from build123d import *

# Parameters (mm, degrees)
SKETCH1_R           = 3.25
SKETCH1_R_2         = 1.5
BOSS_EXTRUDE1_DEPTH = 10


with BuildPart() as part:
    # Sketch1 → Boss-Extrude1 (new body)
    with BuildSketch(Plane(origin=(0, 0, 0), x_dir=(1, 0, 0), z_dir=(0, 1, 0))):
        with BuildLine():
            Line((-40, -26.25), (40, -26.25))
            ThreePointArc((40, -26.25), (44.419417382, -24.419417382), (46.25, -20))
            Line((46.25, -20), (46.25, 20))
            ThreePointArc((46.25, 20), (44.419417382, 24.419417382), (40, 26.25))
            Line((40, 26.25), (-40, 26.25))
            ThreePointArc((-40, 26.25), (-44.419417382, 24.419417382), (-46.25, 20))
            Line((-46.25, 20), (-46.25, -20))
            ThreePointArc((-46.25, -20), (-44.419417382, -24.419417382), (-40, -26.25))
        make_face()
        with Locations((-40, 20)):
            Circle(SKETCH1_R, mode=Mode.SUBTRACT)
        with Locations((-40, -20)):
            Circle(SKETCH1_R, mode=Mode.SUBTRACT)
        with Locations((40, -20)):
            Circle(SKETCH1_R, mode=Mode.SUBTRACT)
        with Locations((40, 20)):
            Circle(SKETCH1_R, mode=Mode.SUBTRACT)
        with Locations((-43.78036994, 13.234550782)):
            Circle(SKETCH1_R_2, mode=Mode.SUBTRACT)
        with Locations((-39.934701703, 12.250275093)):
            Circle(SKETCH1_R_2, mode=Mode.SUBTRACT)
        with Locations((-36.10616509, 13.299212756)):
            Circle(SKETCH1_R_2, mode=Mode.SUBTRACT)
        with Locations((-33.299212756, 16.10616509)):
            Circle(SKETCH1_R_2, mode=Mode.SUBTRACT)
        with Locations((-32.250275093, 19.934701703)):
            Circle(SKETCH1_R_2, mode=Mode.SUBTRACT)
        with Locations((-33.234550782, 23.78036994)):
            Circle(SKETCH1_R_2, mode=Mode.SUBTRACT)
        with Locations((-33.234550782, -23.78036994)):
            Circle(SKETCH1_R_2, mode=Mode.SUBTRACT)
        with Locations((-32.250275093, -19.934701703)):
            Circle(SKETCH1_R_2, mode=Mode.SUBTRACT)
        with Locations((-33.299212756, -16.10616509)):
            Circle(SKETCH1_R_2, mode=Mode.SUBTRACT)
        with Locations((-36.10616509, -13.299212756)):
            Circle(SKETCH1_R_2, mode=Mode.SUBTRACT)
        with Locations((-39.934701703, -12.250275093)):
            Circle(SKETCH1_R_2, mode=Mode.SUBTRACT)
        with Locations((-43.78036994, -13.234550782)):
            Circle(SKETCH1_R_2, mode=Mode.SUBTRACT)
        with Locations((33.234550782, 23.78036994)):
            Circle(SKETCH1_R_2, mode=Mode.SUBTRACT)
        with Locations((32.250275093, 19.934701703)):
            Circle(SKETCH1_R_2, mode=Mode.SUBTRACT)
        with Locations((33.299212756, 16.10616509)):
            Circle(SKETCH1_R_2, mode=Mode.SUBTRACT)
        with Locations((39.934701703, 12.250275093)):
            Circle(SKETCH1_R_2, mode=Mode.SUBTRACT)
        with Locations((43.78036994, 13.234550782)):
            Circle(SKETCH1_R_2, mode=Mode.SUBTRACT)
        with Locations((36.10616509, 13.299212756)):
            Circle(SKETCH1_R_2, mode=Mode.SUBTRACT)
        with Locations((33.234550782, -23.78036994)):
            Circle(SKETCH1_R_2, mode=Mode.SUBTRACT)
        with Locations((32.250275093, -19.934701703)):
            Circle(SKETCH1_R_2, mode=Mode.SUBTRACT)
        with Locations((33.299212756, -16.10616509)):
            Circle(SKETCH1_R_2, mode=Mode.SUBTRACT)
        with Locations((36.10616509, -13.299212756)):
            Circle(SKETCH1_R_2, mode=Mode.SUBTRACT)
        with Locations((39.934701703, -12.250275093)):
            Circle(SKETCH1_R_2, mode=Mode.SUBTRACT)
        with Locations((43.78036994, -13.234550782)):
            Circle(SKETCH1_R_2, mode=Mode.SUBTRACT)
    extrude(amount=BOSS_EXTRUDE1_DEPTH)


solid = part.part
The listing builds one solid part. Answer for the finished solid, in the listing's coordinates (mm). Round coordinates to 2 decimals unless told otherwise and drop trailing zeros. Return JSON: item names as keys, results as strings.
Q1. The mould has two halves that part along Z. Classify faces 1 (the face through (-1, 0, 0)), 2 (the face through (-44.47, 4.93, 24.37)), 3 (the face through (31.736, 4.93, 23.714)): released by +Z, released by -Z, zero draft, split by the parting line, or undercut.
Results list:
{"face 1": "zero draft", "face 2": "released by +Z", "face 3": "undercut"}
Q2. Find section A-A, the plane y = 1. State how many separate pieces and enclosed holes the cut face has, plus the area to 3 significant figures.
Results list:
{"separate pieces": "1", "enclosed holes": "28", "area": "4,520 mm2"}
Q3. Find the intervals of material crossed by line 1 along X through (y, z) = (5.5, -20); line 2 along X through (y, z) = (9, -21); line 3 along Z through (x, y) = (41, 8.25), in increasing order. Write a range as from..to.
Results list:
{"line 1": "x = -46.25..-43.25, -36.75..-33.75, -30.75..30.75, 33.75..36.75, 43.25..46.25", "line 2": "x = -46.17..-43.09, -36.91..-33.31, -31.19..31.19, 33.31..36.91, 43.09..46.17", "line 3": "z = -26.17..-23.09, -16.91..-13.31, -11.19..11.19, 13.31..16.91, 23.09..26.17"}
Q4. This flat-tipped pin is pushed along its axis until it touches: pin 1 Ø5 at (x, z) = (-43.78, 13.23) entering from -Y. Where does it stop, or does it pass through?
Results list:
{"pin 1": "stops at y = 0"}
